The figure shows three views and two pictorial views of one solid part (mm, origin at its lowest corner). Answer the questions. Round coordinates to 2 decimals unless told otherwise and drop trailing zeros. Order: outer loops, then holes, each group sorted by start corner. A loop starts at its lowest first (then second) coordinate and runs counter-clockwise, first axis right, second up. Notation, with made-up numbers: (-30, 53.5) - (-16, 53.5) arc R14 ccw to (-16, 63.5) - close; hole circle Ø3 at (-35.75, 85). An arc over 180 degrees is marked (long way). Write item = value, one per line.
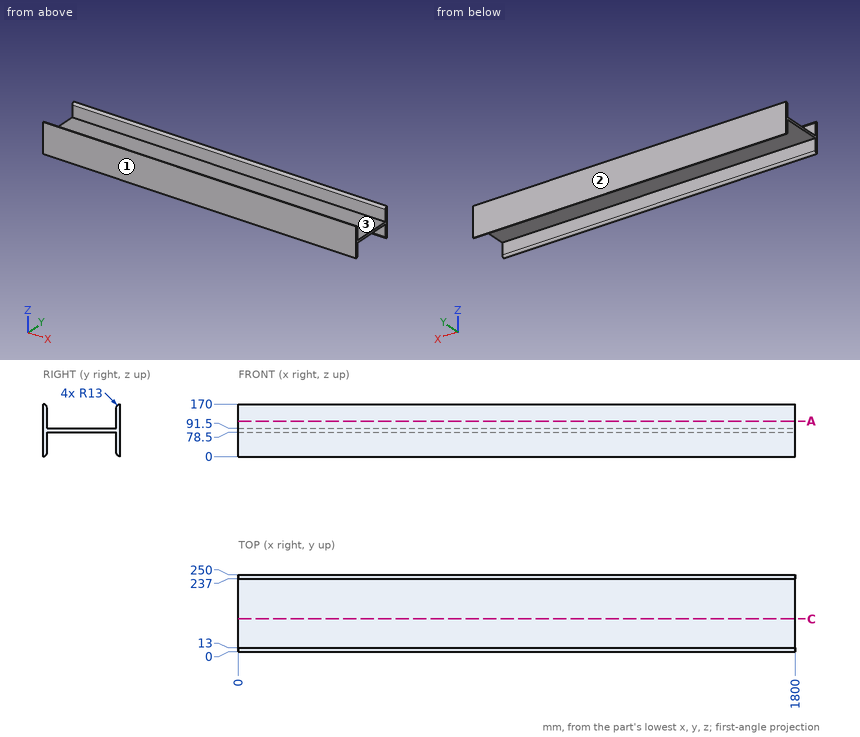
Q1. Section A-A on z = 115 is taken. Determine the outline of the cut face in (x, y), then the cut area to 3 significant figures.
Model answer:
outline = (0, 0) - (1800, 0) - (1800, 13) - (0, 13) - close; (0, 237) - (1800, 237) - (1800, 250) - (0, 250) - close
area = 46,800 mm^2
Q2. Flat-ended cylindrical pins translate along their axes: P1, Ø2, axis at x = 240.5, y = 95, coming from the +Z side; P2, Ø2, axis at x = 860, y = 58, coming from the -Z side. Find the tip coordinate at first contact, or state that the pin passes through.
Model answer:
P1 = 91.5
P2 = 78.5
Q3. Section C-C on y = 107 is taken. Determine the outline of the cut face in (x, z), then the cut area to 3 significant figures.
Model answer:
outline = (0, 78.5) - (1800, 78.5) - (1800, 91.5) - (0, 91.5) - close
area = 23,400 mm^2
Q4. Find the intervals of material crossed by line 1 (Y direction, x = 1163.5, z = 98); line 2 (Z direction, x = 1362.5, y = 174), in increasing order. Write a range as from..to.
Model answer:
line_1 = 0..13, 237..250
line_2 = 78.5..91.5
Q5. Determine the mould class of the marked faces 1, 2 and 3 for opening direction Y: released by +Y, released by -Y, zero draft, split by the parting line, or undercut.
Model answer:
face_1 = released by -Y
face_2 = released by +Y
face_3 = undercut
